For this review, take the finished solid that the model builds, in its own axes (mm). Face numbers are marked on the shaded views. A direction names the side the tool comes from. Round coordinates to 2 decimals unless told otherwise and drop trailing zeros. Order: outer loops, then holes, each group sorted by start corner. A loop starts at its lowest first (then second) coordinate and runs counter-clockwise, first axis right, second up. Notation, with made-up numbers: (-13.5, 36.25) -> (18.5, 36.25) arc R10 cw to (18.5, 40.25) -> close; hole circle Ø3 at (33, -34.75). An arc over 180 degrees is marked (long way). Answer in a Markdown table with one row per item.
```python
from build123d import *

# Parameters (mm, degrees)
SKETCH_1_W               = 65.868
SKETCH_1_H               = 56.896
EXTRUDE_1_DEPTH          = 2
CUT_EXTRUDE_1_DEPTH      = 86.409420089
CUT_EXTRUDE_1_DEPTH_BACK = 86.409420089
SKETCH_3_W               = 2
SKETCH_3_H               = 56.896
EXTRUDE_2_DEPTH          = 18.113
SKETCH_4_W               = 65.868
SKETCH_4_H               = 56.896
EXTRUDE_3_DEPTH          = 2
SKETCH_5_W               = 65.868
SKETCH_5_H               = 20.113
EXTRUDE_4_DEPTH          = 2
FILLET_1_R               = 5
CUT_EXTRUDE_2_DEPTH      = 89.403664002
CUT_EXTRUDE_2_DEPTH_BACK = 89.403664002
SKETCH_6_R               = 4


with BuildPart() as part:
    # Эскиз1 → Бобышка-Вытянуть1 (new body)
    with BuildSketch(Plane(origin=(0, 0, -15.113), x_dir=(-1, 0, 0), z_dir=(0, 0, -1))):
        with Locations((-30.734, 28.448)):
            Rectangle(SKETCH_1_W, SKETCH_1_H)
    extrude(amount=EXTRUDE_1_DEPTH)

    # Эскиз2 → Вырез-Вытянуть1 (cut, two sides: drawn at the far end of the back side and taken through both)
    with BuildSketch(Plane(origin=(0, 0, -17.113), x_dir=(-1, 0, 0), z_dir=(0, 0, -1)).offset(-CUT_EXTRUDE_1_DEPTH_BACK)):
        Polygon((-20.084, 40.396), (-1.8, 40.396), (-1.8, 28.396), (-20.084, 28.396), (-24.084, 28.396), (-24.084, 40.396), align=None)
    extrude(amount=CUT_EXTRUDE_1_DEPTH + CUT_EXTRUDE_1_DEPTH_BACK, mode=Mode.SUBTRACT)

    # Эскиз3 → Бобышка-Вытянуть2 (add)
    with BuildSketch(Plane.XY.offset(-15.113)):
        with Locations((-1.2, 28.448)):
            Rectangle(SKETCH_3_W, SKETCH_3_H)
        with Locations((62.668, 28.448)):
            Rectangle(SKETCH_3_W, SKETCH_3_H)
    extrude(amount=EXTRUDE_2_DEPTH)

    # Эскиз4 → Бобышка-Вытянуть3 (add)
    with BuildSketch(Plane.XY.offset(3)):
        with Locations((30.734, 28.448)):
            Rectangle(SKETCH_4_W, SKETCH_4_H)
    extrude(amount=-EXTRUDE_3_DEPTH)

    # Эскиз5 → Бобышка-Вытянуть4 (add)
    with BuildSketch(Plane(origin=(0, 56.896, 0), x_dir=(1, 0, 0), z_dir=(0, 1, 0))):
        with Locations((30.734, 7.0565)):
            Rectangle(SKETCH_5_W, SKETCH_5_H)
    extrude(amount=EXTRUDE_4_DEPTH)

    # Скругление1
    fillet_1_edges = [part.edges().sort_by_distance(p)[0] for p in [
        (-2.2, 29.448, 3),
        (63.668, 29.448, 3),
        (61.668, 28.448, 1),
        (-0.2, 28.448, 1),
    ]]
    fillet(fillet_1_edges, radius=FILLET_1_R)

    # Эскиз6 → Вырез-Вытянуть2 (cut, two sides: drawn at the far end of the back side and taken through both)
    with BuildSketch(Plane(origin=(0, 58.896, 0), x_dir=(1, 0, 0), z_dir=(0, 1, 0)).offset(-CUT_EXTRUDE_2_DEPTH_BACK)):
        with Locations(Location((9.8, 9.113, 0), (0, 0, 180))):
            Circle(SKETCH_6_R)
    extrude(amount=CUT_EXTRUDE_2_DEPTH + CUT_EXTRUDE_2_DEPTH_BACK, mode=Mode.SUBTRACT)


solid = part.part
```
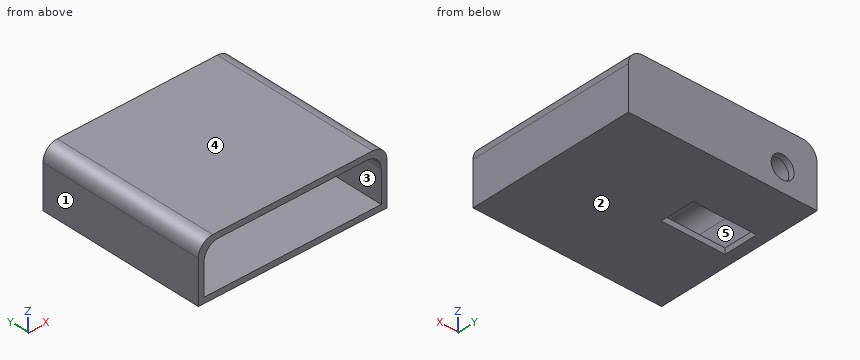
Q1. Take a section at B-B, the plane y = 13. Write out the cut boundary in (x, z), then the cut area to 3 significant figures.
Answer key:
| item | result |
|---|---|
| outline | (-2.2, -17.11) -> (63.67, -17.11) -> (63.67, -2) arc R5 ccw to (58.67, 3) -> (2.8, 3) arc R5 ccw to (-2.2, -2) -> close; hole (-0.2, -15.11) -> (61.67, -15.11) -> (61.67, -4) arc R5 ccw to (56.67, 1) -> (4.8, 1) arc R5 ccw to (-0.2, -4) -> close |
| area | 328 mm^2 |
Q2. Take a section at C-C, the plane x = 18. Write out the cut boundary in (y, z).
Answer key:
| item | result |
|---|---|
| outline | (0, -17.11) -> (28.4, -17.11) -> (28.4, -15.11) -> (0, -15.11) -> close; (0, 1) -> (56.9, 1) -> (56.9, -15.11) -> (40.4, -15.11) -> (40.4, -17.11) -> (58.9, -17.11) -> (58.9, 3) -> (0, 3) -> close |
Q3. Clearance check with flat-ended pins moving along their axes: pin 1 Ø4 at (x, z) = (41.5, -8) entering from -Y; pin 2 Ø5 at (x, z) = (9.8, -9.113) entering from -Y. State where each tip first meets the part, or that it passes through.
Answer key:
| item | result |
|---|---|
| pin 1 | stops at y = 56.9 |
| pin 2 | passes through |
Q4. Tool access review of the marked faces 4 and 5: name each direction out of +Z, -Z, +X, -X, +Y, -Y from which nothing blocks a thin tool from reaching the whole face with its end or side.
Answer key:
| item | result |
|---|---|
| face 4 | +Z, +X, -X, +Y, -Y |
| face 5 | -Y |
Q5. Take a section at A-A, the plane x = 9.8. Write out the cut boundary in (y, z), then the cut area to 3 significant figures.
Answer key:
| item | result |
|---|---|
| outline | (0, -17.11) -> (28.4, -17.11) -> (28.4, -15.11) -> (0, -15.11) -> close; (0, 1) -> (56.9, 1) -> (56.9, -5.11) -> (58.9, -5.11) -> (58.9, 3) -> (0, 3) -> close; (40.4, -17.11) -> (58.9, -17.11) -> (58.9, -13.11) -> (56.9, -13.11) -> (56.9, -15.11) -> (40.4, -15.11) -> close |
| area | 228 mm^2 |
Q6. Take a section at D-D, the plane z = -10.25. Write out the cut boundary in (x, y) (3 decimals), then the cut area to 3 significant figures.
Answer key:
| item | result |
|---|---|
| outline | (-2.2, 0) -> (-0.2, 0) -> (-0.2, 56.896) -> (5.965, 56.896) -> (5.965, 58.896) -> (-2.2, 58.896) -> close; (13.635, 56.896) -> (61.668, 56.896) -> (61.668, 0) -> (63.668, 0) -> (63.668, 58.896) -> (13.635, 58.896) -> close |
| area | 344 mm^2 |
Q7. To check wall thickness, follow probe 1 along X at (y, z) = (11.5, -14); probe 2 along Z at (x, y) = (44.5, 33); probe 3 along Z at (x, y) = (9.8, 57.9). State the ranges of each line that lie inside material, in increasing order.
Answer key:
| item | result |
|---|---|
| probe 1 | x = -2.2 to -0.2, 61.67 to 63.67 |
| probe 2 | z = -17.11 to -15.11, 1 to 3 |
| probe 3 | z = -17.11 to -13.11, -5.11 to 3 |
Q8. The part is to be moulded in two halves that separate along Z. For the marked faces 1, 2 and 3, say which applies: +Z half, -Z half, draft (parallel to the pull), parting line (faces both ways), or undercut.
Answer key:
| item | result |
|---|---|
| face 1 | draft |
| face 2 | -Z half |
| face 3 | undercut |
